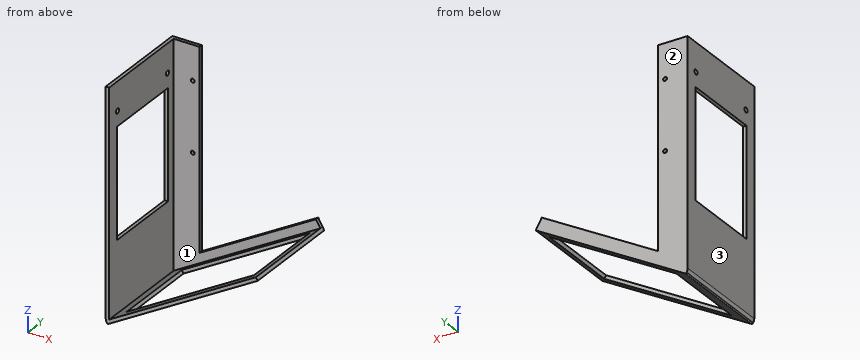
```python
from build123d import *

# Parameters (mm, degrees)
PAD_DEPTH       = 60
SKETCH001_R     = 1.4
SKETCH001_W     = 63
SKETCH001_H     = 46
POCKET_DEPTH    = 2
SKETCH002_W     = 85
SKETCH002_H     = 50
POCKET001_DEPTH = 2.1
SKETCH003_R     = 1.1
PAD001_DEPTH    = 2


with BuildPart() as part:
    # Sketch → Pad (new body)
    with BuildSketch(Plane.XZ):
        with BuildLine():
            Line((2, 130), (0, 130))
            Line((0, 130), (0, 1.092096))
            ThreePointArc((0, 1.092096), (0.138878, 0.037212), (0.546048, -0.945783))
            Line((0.546048, -0.945783), (0.709176, -1.228329))
            ThreePointArc((0.709176, -1.228329), (1.06244, -1.499398), (1.50391, -1.441277))
            Line((87.60254, 48.267949), (1.50391, -1.441277))
            Line((86.60254, 50), (87.60254, 48.267949))
            Line((2, 1.154701), (86.60254, 50))
            Line((2, 1.154701), (2, 130))
        make_face()
    extrude(amount=PAD_DEPTH)

    # Sketch001 (on Face3 of Pad) → Pocket (cut)
    with BuildSketch(Plane(origin=(2, 0, 0), x_dir=(0, 0, 1), z_dir=(1, 0, 0))):
        with Locations((113.5, 52.5)):
            Circle(SKETCH001_R)
        with Locations((113.5, 7.5)):
            Circle(SKETCH001_R)
        with Locations((73.5, 30)):
            Rectangle(SKETCH001_W, SKETCH001_H)
    extrude(amount=-POCKET_DEPTH, mode=Mode.SUBTRACT)

    # Sketch002 (on Face2 of Pocket) → Pocket001 (cut)
    with BuildSketch(Plane(origin=(0, 0, 0), x_dir=(-0.866025, 0, -0.5), z_dir=(-0.5, 0, 0.866025))):
        with Locations((-52.5, 30)):
            Rectangle(SKETCH002_W, SKETCH002_H)
    extrude(amount=-POCKET001_DEPTH, mode=Mode.SUBTRACT)

    # Sketch003 (on Face4 of Pocket001) → Pad001 (join)
    with BuildSketch(Plane(origin=(0, 0, 0), x_dir=(1, 0, 0), z_dir=(0, 1, 0))):
        Polygon((2, -1.154701), (86.60254, -50), (84.10254, -54.330127), (17, -15.588457), (17, -130), (2, -130), align=None)
        with Locations((13, -110)):
            Circle(SKETCH003_R, mode=Mode.SUBTRACT)
        with Locations((13, -70)):
            Circle(SKETCH003_R, mode=Mode.SUBTRACT)
    extrude(amount=-PAD001_DEPTH)


solid = part.part
```
Geometry: final body of the model. Coordinates: model frame, mm. Face numbers are marked on the shaded views. Round coordinates to 2 decimals unless told otherwise and drop trailing zeros. Loops run counter-clockwise (first coordinate to the right, second up) from the corner with the lowest first, then second, coordinate; pieces in that order, holes last.
Item 1: Section C-C, the plane y = -25. Output: boundary loops of the cut face in (x, z).
Checked values:
outline: (0, 1.09) arc R4.08 ccw to (0.55, -0.95) - (0.71, -1.23) arc R0.58 ccw to (1.5, -1.44) - (9.66, 3.27) - (8.66, 5) - (2, 1.15) - (2, 42) - (0, 42) - close; (0, 105) - (2, 105) - (2, 130) - (0, 130) - close; (82.27, 47.5) - (83.27, 45.77) - (87.6, 48.27) - (86.6, 50) - close
Item 2: Section D-D, the plane x = 44. Output: boundary loops of the cut face in (y, z), plus the area to 3 significant figures.
Checked values:
outline: (-60, 23.09) - (-55, 23.09) - (-55, 25.4) - (-60, 25.4) - close; (-5, 23.09) - (0, 23.09) - (0, 31.18) - (-2, 31.18) - (-2, 25.4) - (-5, 25.4) - close
area: 34.6 mm2
Item 3: Section B-B, the plane z = 113.5. Output: boundary loops of the cut face in (x, y), plus the area to 3 significant figures.
Checked values:
outline: (0, -60) - (2, -60) - (2, -53.9) - (0, -53.9) - close; (0, -51.1) - (2, -51.1) - (2, -8.9) - (0, -8.9) - close; (0, -6.1) - (2, -6.1) - (2, -2) - (17, -2) - (17, 0) - (0, 0) - close
area: 139 mm2
Item 4: Section A-A, the plane z = 96. Output: boundary loops of the cut face in (x, y).
Checked values:
outline: (0, -60) - (2, -60) - (2, -53) - (0, -53) - close; (0, -7) - (2, -7) - (2, -2) - (17, -2) - (17, 0) - (0, 0) - close
Item 5: Contact query for flat-ended pins moving along their axis: P1, Ø1, axis at x = 12.5, z = 41, coming from the -Y side; P2, Ø3.5, axis at x = 13, z = 110, coming from the +Y side; P3, Ø17.5, axis at y = -45, z = 58.5, coming from the +X side; P4, Ø2, axis at y = -1, z = 84, coming from the +X side. Output: stop coordinate, or through.
Checked values:
P1: stops at y = -2
P2: stops at y = 0
P3: stops at x = 86.75
P4: stops at x = 17
Item 6: Line query: L1, parallel to Z at x = 0.7, y = -7.5; L2, parallel to Y at x = 1.65, z = 113.5; L3, parallel to X at y = -0.5, z = 110. Output: solid intervals per line, ascending.
Checked values:
L1: z = -1.21 to 42, 105 to 112.1, 114.9 to 130
L2: y = -60 to -53.9, -51.1 to -8.9, -6.1 to 0
L3: x = 0 to 11.9, 14.1 to 17
Item 7: Mould query, pull axis X, two halves, no side actions, for the marked faces 1, 2 and 3. Classes: released by +X, released by -X, zero draft, split by the parting line, or undercut.
Checked values:
face 1: undercut
face 2: zero draft
face 3: released by -X
